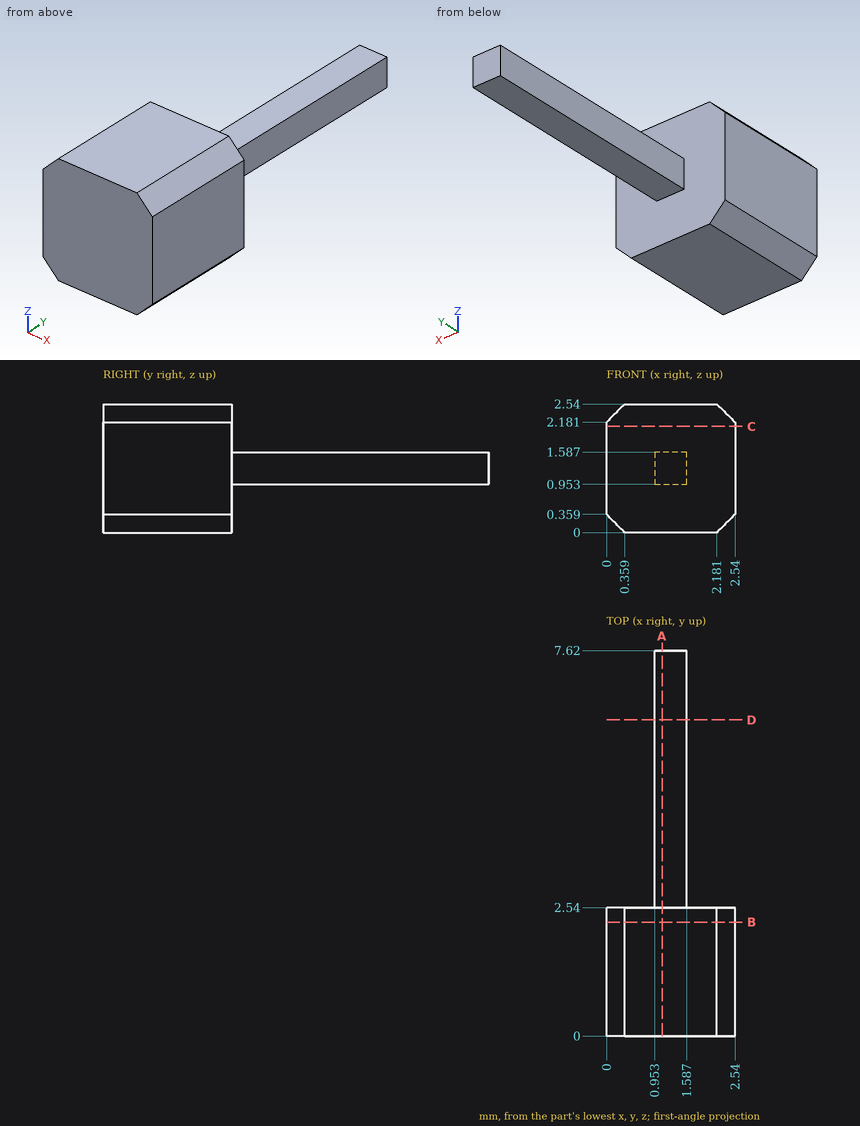
Input: dimensioned drawing with shaded views. Units: mm. Origin: part minimum x, y, z. Give positions to 0.01 mm unless a question says otherwise; leave off trailing zeros. Loops run counter-clockwise (first coordinate to the right, second up) from the corner with the lowest first, then second, coordinate; pieces in that order, holes last. Notation, with made-up numbers: (41.25, -28) -> (96.25, -28) arc R22 cw to (96.25, 9) -> close; hole circle Ø5 at (-7, 48.5). An arc over 180 degrees is marked (long way). Return JSON: item names as keys, results as strings.
Item 1: Pin query (flat end, axial travel): P1, Ø0.5, axis at y = 6, z = 1, coming from the -X side; P2, Ø0.5, axis at y = 4, z = 1.5, coming from the +X side; P3, Ø1, axis at x = 2, y = 5.5, coming from the +Z side. Return the tip coordinate at first contact, or that it passes through.
Filled in:
{"P1": "x = 0.95", "P2": "x = 1.59", "P3": "z = 1.59"}
Item 2: Section D-D, the plane y = 6.25. Output: boundary loops of the cut face in (x, z).
Filled in:
{"outline": "(0.95, 0.95) -> (1.59, 0.95) -> (1.59, 1.59) -> (0.95, 1.59) -> close"}
Item 3: Section B-B, the plane y = 2.25. Output: boundary loops of the cut face in (x, z).
Filled in:
{"outline": "(0, 0.36) -> (0.36, 0) -> (2.18, 0) -> (2.54, 0.36) -> (2.54, 2.18) -> (2.18, 2.54) -> (0.36, 2.54) -> (0, 2.18) -> close"}
Item 4: Section C-C, the plane z = 2.1. Output: boundary loops of the cut face in (x, y).
Filled in:
{"outline": "(0, 0) -> (2.54, 0) -> (2.54, 2.54) -> (0, 2.54) -> close"}
Item 5: Line query: line 1 (Y direction, x = 2.45, z = 0.8); line 2 (Z direction, x = 1.2, y = 3.5). Output: solid intervals per line, ascending.
Filled in:
{"line 1": "0 to 2.54", "line 2": "0.95 to 1.59"}
Item 6: Section A-A, the plane x = 1.1. Output: boundary loops of the cut face in (y, z).
Filled in:
{"outline": "(0, 0) -> (2.54, 0) -> (2.54, 0.95) -> (7.62, 0.95) -> (7.62, 1.59) -> (2.54, 1.59) -> (2.54, 2.54) -> (0, 2.54) -> close"}
